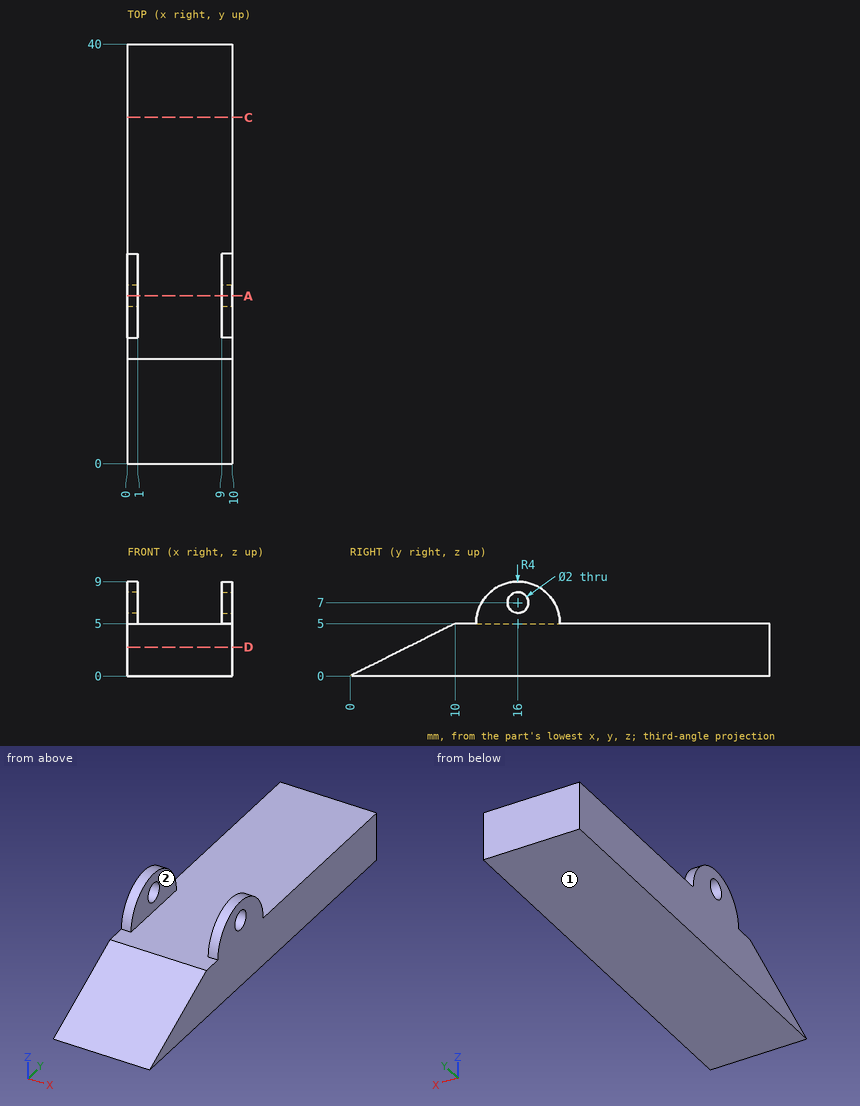
Geometry check sheet. Reference: drawing and pictorial views, mm from the part's lowest x, y, z. A direction names the side the tool comes from. Coordinates: 2 decimals unless noted, no trailing zeros. Loops run counter-clockwise (first coordinate to the right, second up) from the corner with the lowest first, then second, coordinate; pieces in that order, holes last. Notation, with made-up numbers: (44.25, 65.5) -> (68.25, 65.5) arc R24 cw to (68.25, 98.5) -> close; hole circle Ø2 at (56, 3.5). An arc over 180 degrees is marked (long way). Write item = value, one per line. Start each with the question number.
1. Material ranges on line 1 (Z direction, x = 0.55, y = 16); line 2 (X direction, y = 13, z = 7.5); line 3 (Y direction, x = 6, z = 3), recorded low to high.
2. Tool access check on the marked faces 1 and 2. Record the directions out of +Z, -Z, +X, -X, +Y, -Y that give a thin tool (end or side, any length) a straight path to the whole face; none if there is none.
3. Section check D-D on z = 2.75. Record the cut outline in (x, y).
4. Section check A-A on y = 16. Record the cut outline in (x, z), then the cut area to 3 significant figures.
5. Depth check by flat-ended pin: P1, Ø3, axis at x = 5.5, z = 7.5, coming from the -Y side; P2, Ø5, axis at x = 5.5, y = 19, coming from the +Z side; P3, Ø5, axis at x = 7, z = 8, coming from the +Y side; P4, Ø6, axis at x = 6.5, y = 20, coming from the +Z side. Enter the tip coordinate at first touch or a pass-through.
6. Section check C-C on y = 33. Record the cut outline in (x, z).
Responses:
q1.line_1 = 0 to 6, 8 to 9
q1.line_2 = 0 to 1, 9 to 10
q1.line_3 = 6 to 40
q2.face_1 = -Z, +X, -X, +Y, -Y
q2.face_2 = +Z, +Y, -Y
q3.outline = (0, 5.5) -> (10, 5.5) -> (10, 40) -> (0, 40) -> close
q4.outline = (0, 0) -> (10, 0) -> (10, 6) -> (9, 6) -> (9, 5) -> (1, 5) -> (1, 6) -> (0, 6) -> close; (0, 8) -> (1, 8) -> (1, 9) -> (0, 9) -> close; (9, 8) -> (10, 8) -> (10, 9) -> (9, 9) -> close
q4.area = 54.0 mm2
q5.P1 = through
q5.P2 = 5
q5.P3 = 19.71
q5.P4 = 8.24
q6.outline = (0, 0) -> (10, 0) -> (10, 5) -> (0, 5) -> close
